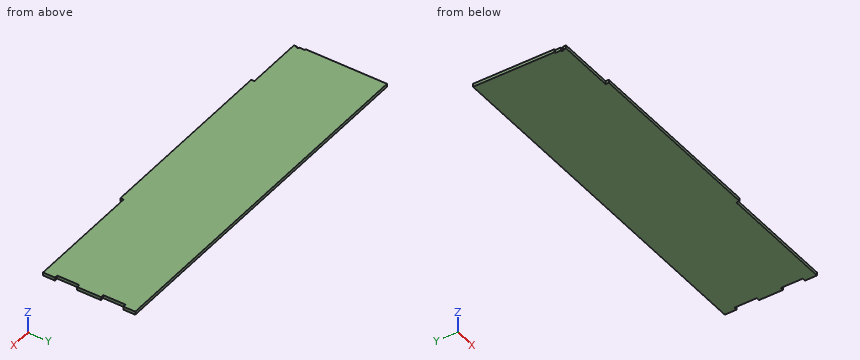
```python
from build123d import *

# Parameters (mm, degrees)
SALIENTE_EXTRUIR1_DEPTH = 5
CROQUIS2_W              = 5
CROQUIS2_H              = 35
CORTAR_EXTRUIR1_DEPTH   = 5
CORTAR_EXTRUIR2_DEPTH   = 10
CORTAR_EXTRUIR5_DEPTH   = 10


with BuildPart() as part:
    # Croquis1 → Saliente-Extruir1 (new body)
    with BuildSketch(Plane.XY):
        Polygon((0, 145), (0, 0), (183.734642654, 0), (185, 0), (185, -5), (485, -5), (485, 0), (670, 0), (670, -5), (970, -5), (970, 0), (1155, 0), (1155, -5), (1455, -5), (1455, 0), (1640, 0), (1640, 145), align=None)
    extrude(amount=SALIENTE_EXTRUIR1_DEPTH)

    # Croquis2 → Cortar-Extruir1 (cut)
    with BuildSketch(Plane.XY.offset(5)):
        with Locations((1637.5, 108.75)):
            Rectangle(CROQUIS2_W, CROQUIS2_H)
        with Locations((1637.5, 36.25)):
            Rectangle(CROQUIS2_W, CROQUIS2_H)
        with Locations((2.5, 36.25)):
            Rectangle(CROQUIS2_W, CROQUIS2_H)
        with Locations((2.5, 108.75)):
            Rectangle(CROQUIS2_W, CROQUIS2_H)
    extrude(amount=-CORTAR_EXTRUIR1_DEPTH, mode=Mode.SUBTRACT)

    # Croquis3 → Cortar-Extruir2 (cut)
    with BuildSketch(Plane.XY.offset(5)):
        Polygon((579.3, 0), (575.7, 0), (575.7, 5), (573.9, 5), (573.9, 8.2), (575.7, 8.2), (575.7, 17.2), (579.3, 17.2), (579.3, 8.2), (581.1, 8.2), (581.1, 5), (579.3, 5), align=None)
        Polygon((1064.3, 8.2), (1064.3, 17.2), (1060.7, 17.2), (1060.7, 8.2), (1058.9, 8.2), (1058.9, 5), (1060.7, 5), (1060.7, 0), (1064.3, 0), (1064.3, 5), (1066.1, 5), (1066.1, 8.2), align=None)
    extrude(amount=-CORTAR_EXTRUIR2_DEPTH, mode=Mode.SUBTRACT)

    # Croquis4 → Cortar-Extruir5 (cut)
    with BuildSketch(Plane.XY.offset(5)):
        Polygon((1062.5, 17.2), (1062.5, 145), (0, 145), (0, -10.556117746), (1062.5, -10.556117746), align=None)
    extrude(amount=-CORTAR_EXTRUIR5_DEPTH, mode=Mode.SUBTRACT)


solid = part.part
```
Geometry: final body of the model. Coordinates: model frame, mm. Coordinates: 2 decimals unless noted, no trailing zeros. Order: outer loops, then holes, each group sorted by start corner. A loop starts at its lowest first (then second) coordinate and runs counter-clockwise, first axis right, second up. Notation, with made-up numbers: (-36.75, -16) -> (-7.75, -16) arc R11 ccw to (-7.75, -6) -> close; hole circle Ø9 at (76, -25.5). An arc over 180 degrees is marked (long way). Use CSV: the item, a comma, the result in double quotes.
1) Pin query (flat end, axial travel): pin 1 Ø0.5 at (x, z) = (1063.5, 2.5) entering from -Y; pin 2 Ø2 at (x, z) = (1065, 2) entering from -Y; pin 3 Ø2.5 at (y, z) = (105, 3.5) entering from +X. Return the tip coordinate at first contact, or that it passes through.
Findings:
pin 1,"stops at y = 17.2"
pin 2,"stops at y = 0"
pin 3,"stops at x = 1635"
2) Section A-A on z = 1.25. Output: boundary loops of the cut face in (x, y).
Findings:
outline,"(1062.5, 17.2) -> (1064.3, 17.2) -> (1064.3, 8.2) -> (1066.1, 8.2) -> (1066.1, 5) -> (1064.3, 5) -> (1064.3, 0) -> (1155, 0) -> (1155, -5) -> (1455, -5) -> (1455, 0) -> (1640, 0) -> (1640, 18.75) -> (1635, 18.75) -> (1635, 53.75) -> (1640, 53.75) -> (1640, 91.25) -> (1635, 91.25) -> (1635, 126.25) -> (1640, 126.25) -> (1640, 145) -> (1062.5, 145) -> close"
3) Section B-B on x = 1542. Output: boundary loops of the cut face in (y, z), then the cut area to 3 significant figures.
Findings:
outline,"(0, 0) -> (145, 0) -> (145, 5) -> (0, 5) -> close"
area,"725 mm^2"
4) Line query: line 1 (X direction, y = 41, z = 3.75); line 2 (Y direction, x = 1472.5, z = 2.3). Output: solid intervals per line, ascending.
Findings:
line 1,"x = 1062.5 to 1635"
line 2,"y = 0 to 145"
